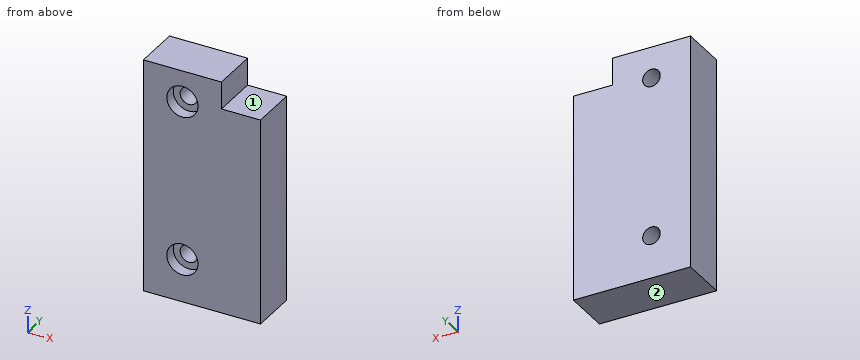
from build123d import *

# Parameters (mm, degrees)
F0_R     = 2.25
F1_DEPTH = 12
F2_R     = 4
F2_R_2   = 2.25
F3_DEPTH = 3


with BuildPart() as f1:
    # F0 (on Front) → F1 (new body)
    with BuildSketch(Plane.XZ):
        Polygon((0, 60), (0, 0), (30, 0), (30, 53), (20, 53), (20, 60), align=None)
        with Locations((10, 11)):
            Circle(F0_R, mode=Mode.SUBTRACT)
        with Locations((10, 52)):
            Circle(F0_R, mode=Mode.SUBTRACT)
    extrude(amount=F1_DEPTH)

    # F2 (on face) → F3 (cut)
    with BuildSketch(Plane.XZ.offset(12)):
        with Locations((10, 52)):
            Circle(F2_R)
        with Locations((10, 52)):
            Circle(F2_R_2, mode=Mode.SUBTRACT)
        with Locations((10, 11)):
            Circle(F2_R)
        with Locations((10, 11)):
            Circle(F2_R_2, mode=Mode.SUBTRACT)
    extrude(amount=-F3_DEPTH, mode=Mode.SUBTRACT)


solid = f1.part
Here's how the part is built. I have some questions about the finished solid (model axes, mm). Face numbers are marked on the shaded views. A direction names the side the tool comes from. Coordinates: 2 decimals unless noted, no trailing zeros. Order: outer loops, then holes, each group sorted by start corner. A loop starts at its lowest first (then second) coordinate and runs counter-clockwise, first axis right, second up. Notation, with made-up numbers: (51.5, -4.75) -> (60.5, -4.75) arc R33 ccw to (60.5, 33.25) -> close; hole circle Ø2 at (87, 38.25). An arc over 180 degrees is marked (long way). Answer in a Markdown table with one row per item.
(1) On a 3-axis mill with a long thin cutter (end or side, diameter ignored), from which of +Z, -Z, +X, -X, +Y, -Y can I reach the whole of each face in a straight line? I mean the marked faces 1 and 2. Say none if no direction works.
Answer key:
| item | result |
|---|---|
| face 1 | +Z, +X, +Y, -Y |
| face 2 | -Z, +X, -X, +Y, -Y |
(2) I want a section at C-C on y = -7. List the corners of the cut face in (x, z) for me.
Answer key:
| item | result |
|---|---|
| outline | (0, 0) -> (30, 0) -> (30, 53) -> (20, 53) -> (20, 60) -> (0, 60) -> close; hole circle Ø4.5 at (10, 11); hole circle Ø4.5 at (10, 52) |
(3) I want a section at A-A on x = 10. List the corners of the cut face in (y, z) for me.
Answer key:
| item | result |
|---|---|
| outline | (-12, 0) -> (0, 0) -> (0, 8.75) -> (-9, 8.75) -> (-9, 7) -> (-12, 7) -> close; (-12, 15) -> (-9, 15) -> (-9, 13.25) -> (0, 13.25) -> (0, 49.75) -> (-9, 49.75) -> (-9, 48) -> (-12, 48) -> close; (-12, 56) -> (-9, 56) -> (-9, 54.25) -> (0, 54.25) -> (0, 60) -> (-12, 60) -> close |
(4) I want a section at D-D on z = 12.5. List the corners of the cut face in (x, y) for me.
Answer key:
| item | result |
|---|---|
| outline | (0, -12) -> (6.29, -12) -> (6.29, -9) -> (8.32, -9) -> (8.32, 0) -> (0, 0) -> close; (11.68, -9) -> (13.71, -9) -> (13.71, -12) -> (30, -12) -> (30, 0) -> (11.68, 0) -> close |
(5) Please list where these lines run through material, in increasing order: probe 1 along Z at (x, y) = (10, -10.1); probe 2 along Z at (x, y) = (10, -3.25); probe 3 along Y at (x, z) = (10.5, 13.5).
Answer key:
| item | result |
|---|---|
| probe 1 | 0 to 7, 15 to 48, 56 to 60 |
| probe 2 | 0 to 8.75, 13.25 to 49.75, 54.25 to 60 |
| probe 3 | -9 to 0 |
(6) Will these pins go through, and if not, where does the flat tip stop? pin 1 Ø3.5 at (x, z) = (10, 52) entering from -Y; pin 2 Ø2.5 at (x, z) = (11.5, 50.5) entering from -Y; pin 3 Ø5 at (x, y) = (26, -3.5) entering from +Z; pin 4 Ø3.5 at (y, z) = (-6.5, 57.5) entering from +X.
Answer key:
| item | result |
|---|---|
| pin 1 | through |
| pin 2 | y = -9 |
| pin 3 | z = 53 |
| pin 4 | x = 20 |
(7) I want a section at B-B on z = 52. List the corners of the cut face in (x, y) for me, then the cut area to 4 significant figures.
Answer key:
| item | result |
|---|---|
| outline | (0, -12) -> (6, -12) -> (6, -9) -> (7.75, -9) -> (7.75, 0) -> (0, 0) -> close; (12.25, -9) -> (14, -9) -> (14, -12) -> (30, -12) -> (30, 0) -> (12.25, 0) -> close |
| area | 295.5 mm^2 |
